Can you work these out from the model? Positions are in its coordinate system, mm. A direction names the side the tool comes from. Round coordinates to 2 decimals unless told otherwise and drop trailing zeros. Loops run counter-clockwise (first coordinate to the right, second up) from the corner with the lowest first, then second, coordinate; pieces in that order, holes last. Notation, with made-up numbers: (3.25, -9) -> (60.25, -9) arc R14 ccw to (60.25, 10) -> close; hole circle Ø7 at (-9, 87). An arc over 180 degrees is marked (long way). Write each question's results on one line, items separated by ' | '.
from build123d import *

# Parameters (mm, degrees)
F1_DEPTH = 6.35
F2_DEPTH = 6.35
F0_R     = 10.7670897693
F5_DEPTH = 6.35
F6_D     = 6.35


# Not quite as in the source:
# - a feature of the source that left no trace in its solid (it failed there, or was rolled back) is left out


with BuildPart() as f1:
    # F0 (on Right) → F1 (new body)
    with BuildSketch(Plane.YZ):
        with BuildLine():
            ThreePointArc((-1.5825573364, -153.9491721496), (-1.5826429755, -154.035180638), (-1.5828998925, -154.1211887854))
            Line((-1.5828998925, -154.1211887854), (13.683948877, -58.1386835494))
            ThreePointArc((13.683948877, -58.1386835494), (37.0236297514, -16.510860014), (81.800944289, 0))
            Line((81.800944289, 0), (125.0803981306, 0))
            ThreePointArc((125.0803981306, 0), (149.2715136598, -6.5386249673), (166.8746197449, -24.3738245223))
            Line((166.8746197449, -24.3738245223), (187.8910975974, -61.5208026845))
            ThreePointArc((187.8910975974, -61.5208026845), (190.6720383022, -62.6941019502), (192.5146989034, -60.3035237191))
            Line((192.5146989034, -60.3035237191), (192.5146989034, -2.1215420715))
            Line((192.5146989034, -2.1215420715), (198.7226175975, 77.2382490494))
            ThreePointArc((198.7226175975, 77.2382490494), (197.2700771229, 79.4482102797), (194.7679715475, 78.5918983278))
            Line((194.7679715475, 78.5918983278), (171.5573410493, 43.2821044094))
            ThreePointArc((171.5573410493, 43.2821044094), (155.3522029023, 29.6366600871), (134.3221352203, 27.0791405068))
            Line((134.3221352203, 27.0791405068), (-15.8528228172, 52.6105930486))
            ThreePointArc((-15.8528228172, 52.6105930486), (-33.2247403603, 48.9627075804), (-43.4379661828, 34.4444223576))
            Line((-43.4379661828, 34.4444223576), (-85.8287484087, -140.5429926023))
            ThreePointArc((-85.8287484087, -140.5429926023), (-37.9848929099, -111.2960762471), (-1.5825573364, -153.9491721496))
        make_face()
    extrude(amount=F1_DEPTH)

    # F0 (on Right) → F2 (join)
    with BuildSketch(Plane.YZ):
        with BuildLine():
            ThreePointArc((-1.5825573364, -153.9491721496), (-1.5826429755, -154.035180638), (-1.5828998925, -154.1211887854))
            Line((-1.5828998925, -154.1211887854), (13.683948877, -58.1386835494))
            ThreePointArc((13.683948877, -58.1386835494), (37.0236297514, -16.510860014), (81.800944289, 0))
            Line((81.800944289, 0), (125.0803981306, 0))
            ThreePointArc((125.0803981306, 0), (149.2715136598, -6.5386249673), (166.8746197449, -24.3738245223))
            Line((166.8746197449, -24.3738245223), (187.8910975974, -61.5208026845))
            ThreePointArc((187.8910975974, -61.5208026845), (190.6720383022, -62.6941019502), (192.5146989034, -60.3035237191))
            Line((192.5146989034, -60.3035237191), (192.5146989034, -2.1215420715))
            Line((192.5146989034, -2.1215420715), (198.7226175975, 77.2382490494))
            ThreePointArc((198.7226175975, 77.2382490494), (197.2700771229, 79.4482102797), (194.7679715475, 78.5918983278))
            Line((194.7679715475, 78.5918983278), (171.5573410493, 43.2821044094))
            ThreePointArc((171.5573410493, 43.2821044094), (155.3522029023, 29.6366600871), (134.3221352203, 27.0791405068))
            Line((134.3221352203, 27.0791405068), (-15.8528228172, 52.6105930486))
            ThreePointArc((-15.8528228172, 52.6105930486), (-33.2247403603, 48.9627075804), (-43.4379661828, 34.4444223576))
            Line((-43.4379661828, 34.4444223576), (-85.8287484087, -140.5429926023))
            ThreePointArc((-85.8287484087, -140.5429926023), (-37.9848929099, -111.2960762471), (-1.5825573364, -153.9491721496))
        make_face()
    extrude(amount=F2_DEPTH)

    # F0 (on Right) → F5 (join)
    with BuildSketch(Plane.YZ):
        with BuildLine():
            ThreePointArc((-85.8287484087, -140.5429926023), (-51.6446777228, -196.588666929), (-1.5828998925, -154.1211887854))
            ThreePointArc((-1.5828998925, -154.1211887854), (-1.5826429755, -154.035180638), (-1.5825573364, -153.9491721496))
            ThreePointArc((-1.5825573364, -153.9491721496), (-37.9848929099, -111.2960762471), (-85.8287484087, -140.5429926023))
        make_face()
        with Locations((-44.772322165, -153.9491721496)):
            Circle(F0_R, mode=Mode.SUBTRACT)
    extrude(amount=F5_DEPTH)

    # F6 (through all)
    with Locations(Plane(origin=(0, 0, 0), x_dir=(0, 1, 0), z_dir=(-1, 0, 0))):
        with Locations((-44.772322165, 130.1366721496), (-24.1500922374, 142.0429221496), (-24.1500922374, 165.8554221496), (-44.772322165, 177.7616721496), (-65.3945520927, 165.8554221496), (-65.3945520927, 142.0429221496)):
            Hole(F6_D / 2)


solid = f1.part
1. If we section it at C-C (z = -36): List the corners of the cut face in (x, y) for me.
Final values:
outline: (0, -60.5) -> (6.35, -60.5) -> (6.35, 21.22) -> (0, 21.22) -> close; (0, 173.45) -> (6.35, 173.45) -> (6.35, 192.51) -> (0, 192.51) -> close
2. Please list where these lines run through material, in increasing order: line 1 (Y direction, x = 0.5, z = -26); line 2 (Y direction, x = 5.25, z = -12); line 3 (Z direction, x = 1.5, y = 132). Write a range as from..to.
Final values:
line 1: -58.08..27.85, 167.79..192.51 | line 2: -54.69..42.92, 156.84..192.51 | line 3: -0.5..27.47
3. If we section it at B-B (x = 1.75): List the corners of the cut face in (y, z) for me (3 decimals), then the cut area to 3 significant figures.
Final values:
outline: (-85.829, -140.543) arc R43.19 ccw (long way) to (-1.583, -154.121) -> (13.684, -58.139) arc R68.973 cw to (81.801, 0) -> (125.08, 0) arc R48.02 cw to (166.875, -24.374) -> (187.891, -61.521) arc R2.472 ccw to (192.515, -60.304) -> (192.515, -2.122) -> (198.723, 77.238) arc R2.158 ccw to (194.768, 78.592) -> (171.557, 43.282) arc R37.115 cw to (134.322, 27.079) -> (-15.853, 52.611) arc R24.208 ccw to (-43.438, 34.444) -> close; hole circle Ø6.35 at (-65.395, -165.855); hole circle Ø6.35 at (-65.395, -142.043); hole circle Ø21.534 at (-44.772, -153.949); hole circle Ø6.35 at (-44.772, -177.762); hole circle Ø6.35 at (-44.772, -130.137); hole circle Ø6.35 at (-24.15, -165.855); hole circle Ø6.35 at (-24.15, -142.043) | area: 27,200 mm2
4. If we section it at D-D (y = 55): List the corners of the cut face in (x, z) for me, then the cut area to 3 significant figures.
Final values:
outline: (0, -5.42) -> (6.35, -5.42) -> (6.35, 40.56) -> (0, 40.56) -> close | area: 292 mm2
5. On a 3-axis mill with a long thin cutter (end or side, diameter ignored), from which of +Z, -Z, +X, -X, +Y, -Y can I reach the whole of each face in a straight line? I mean faces 4 (the face through (3.131, -64.337, -51.824)), 5 (the face through (3.131, 183.325, 61.184)), 6 (the face through (3.13, 148.96, -6.36)). Say none if no direction works.
Final values:
face 4: +Z, +X, -X, -Y | face 5: +Z, +X, -X | face 6: -Z, +X, -X
6. Will these pins go through, and if not, where does the flat tip stop? pin 1 (3 mm diameter, centred on x = 3, y = 105, fed in from -Z); pin 2 (2 mm diameter, centred on x = 1.5, z = -161, fed in from -Y); pin 3 (2 mm diameter, centred on x = 5, z = -69, fed in from +Y).
Final values:
pin 1: z = 0 | pin 2: y = -87.54 | pin 3: y = 12.12
7. We'd pull the mould along Y, two halves only. Please class faces 1 (the face through (3, 103, 0)), 2 (the face through (3.13, -52.67, -196.41)), 3 (the face through (3, 192.515, -32)): pulls with the +Y half, pulls with the -Y half, needs draft (parallel to the pull), parting line crosses it, or undercut.
Final values:
face 1: undercut | face 2: parting line crosses it | face 3: pulls with the +Y half
8. If we section it at A-A (z = 31): List the corners of the cut face in (x, y) for me.
Final values:
outline: (0, -44.27) -> (6.35, -44.27) -> (6.35, 111.26) -> (0, 111.26) -> close; (0, 158.16) -> (6.35, 158.16) -> (6.35, 195.11) -> (0, 195.11) -> close
